Design review of the part built by this model. Coordinates are the model's own, in mm. A direction names the side the tool comes from. Coordinates: 2 decimals unless noted, no trailing zeros. Order: outer loops, then holes, each group sorted by start corner. A loop starts at its lowest first (then second) coordinate and runs counter-clockwise, first axis right, second up. Notation, with made-up numbers: (49.5, 11) -> (98.5, 11) arc R34 cw to (98.5, 41) -> close; hole circle Ø2 at (32.25, 79.5). An arc over 180 degrees is marked (long way). Use a Markdown table: item, result. Add a question column.
Q1. Add section C-C (z = 4). State the section outline as (x, y) points, then the cut area to 3 significant figures.
Q2. Machinability: for faces 1 (the face through (7.62, -3.16, 4.54)), 2 (the face through (-7, -5, 7)), 3 (the face through (-2.17, -9.76, 3.48)), which of the approach directions +Z, -Z, +X, -X, +Y, -Y give a long, thin tool a straight path to every point of the face, cutting with its end or side? Answer none if there is none.
Q3. Wall thickness on probe 1 along Y at (x, z) = (0, 3.4); probe 2 along Z at (x, y) = (2, -6); probe 3 along Y at (x, z) = (-5.5, 9.5): over which ranges is each line inside the solid? List them lowest first.
Q4. Insertion check: pin 1 (6 mm diameter, centred on x = -5.5, z = 3, fed in from +Y); pin 2 (4 mm diameter, centred on y = -3.5, z = 7.5, fed in from -X); pin 3 (2 mm diameter, centred on x = 1, z = 9, fed in from -Y). Each pin has a flat end and moves straight along its axis. Give the tip position at first contact, or say it passes through.
Q5. Add section A-A (y = 0). State the section outline as (x, z) points (3 decimals), then the cut area to 3 significant figures.
Q6. Add section D-D (z = 6). State the section outline as (x, y) points.
Q7. The part is to be moulded in two halves that separate along X. For faces 4 (the face through (4.449, -8.554, 8.576)), 5 (the face through (-1.978, -8.908, 8.331)), 6 (the face through (0, 0, 0)), say which applies: pulls with the +X half, pulls with the -X half, needs draft (parallel to the pull), parting line crosses it, or undercut.
from build123d import *

# Parameters (mm, degrees)
F0_R        = 10
F1_DEPTH    = 10
F2_R        = 8.25
F3_DEPTH    = 8
F4_R        = 9.125
F4_R_2      = 8.25
F5_DEPTH    = 3
F6_R        = 9.125
F6_R_2      = 8.75
F7_DEPTH    = 1
F8_R        = 2
F9_S5_R     = 9.125
F9_T6_DEPTH = 15
F10_SIZE2   = 5
F10_SIZE    = 0.5


# Not quite as in the source:
# - a fillet or chamfer that OpenCascade refuses, or shapes differently, is made with other operations: its cross-section is extruded or revolved along the edge and cut away or added


with BuildPart() as f1:
    # F0 (on Top) → F1 (new body)
    with BuildSketch(Plane.XY):
        Circle(F0_R)
    extrude(amount=F1_DEPTH)

    # F2 (on face) → F3 (cut)
    with BuildSketch(Plane.XY.offset(10)):
        Circle(F2_R)
    extrude(amount=-F3_DEPTH, mode=Mode.SUBTRACT)

    # F4 (on face) → F5 (cut)
    with BuildSketch(Plane.XY.offset(10)):
        Circle(F4_R)
        Circle(F4_R_2, mode=Mode.SUBTRACT)
    extrude(amount=-F5_DEPTH, mode=Mode.SUBTRACT)

    # F6 (on face) → F7 (join)
    with BuildSketch(Plane.XY.offset(10)):
        Circle(F6_R)
        Circle(F6_R_2, mode=Mode.SUBTRACT)
    extrude(amount=-F7_DEPTH)

    # F8
    f8_edges = [f1.edges().sort_by_distance(p)[0] for p in [
        (-10, 0, 0),
    ]]
    fillet(f8_edges, radius=F8_R)

    # F9: chamfer of 1 on 1 edges, made by hand


with BuildPart() as f9_tool2:
    # F9_s3 → F9_t4 (revolve)
    with BuildSketch(Plane.XZ):
        Polygon((8.75, 10), (9.75, 9), (8.75, 9), align=None)
    revolve(axis=Axis((0, 0, 9), (0, 0, 1)))

    # F9_s5 → F9_t6 (intersect, symmetric)
    with BuildSketch(Plane.XY.offset(9.5)):
        Circle(F9_S5_R)
    extrude(amount=F9_T6_DEPTH, both=True, mode=Mode.INTERSECT)


with BuildPart() as f1_1:
    add(f1.part)

    # F9_t1: cut F9_tool2
    add(f9_tool2.part, mode=Mode.SUBTRACT)

    # F10
    f10_edges = [f1_1.edges().sort_by_distance(p)[0] for p in [
        (-10, 0, 10),
    ]]
    f10_side = f1_1.faces().sort_by_distance((-9.717157, 0, 10))[0]
    chamfer(f10_edges, length=F10_SIZE, length2=F10_SIZE2, reference=f10_side)


solid = f1_1.part
Established:
| question | item | result |
|---|---|---|
| 1 | outline | circle Ø20 at (0, 0); hole circle Ø16.5 at (0, 0) |
| 1 | area | 100 mm^2 |
| 2 | face 1 | +Z |
| 2 | face 2 | none |
| 2 | face 3 | +Z, -Z |
| 3 | probe 1 | -10 to -8.25, 8.25 to 10 |
| 3 | probe 2 | 0 to 2 |
| 3 | probe 3 | -7.81 to -7.28, 7.28 to 7.81 |
| 4 | pin 1 | y = 9.68 |
| 4 | pin 2 | x = -9.69 |
| 4 | pin 3 | y = -9.67 |
| 5 | outline | (-10, 2) arc R2 ccw to (-8, 0) -> (8, 0) arc R2 ccw to (10, 2) -> (10, 5) -> (9.5, 10) -> (8.75, 10) -> (9.125, 9.625) -> (9.125, 7) -> (8.25, 7) -> (8.25, 2) -> (-8.25, 2) -> (-8.25, 7) -> (-9.125, 7) -> (-9.125, 9.625) -> (-8.75, 10) -> (-9.5, 10) -> (-10, 5) -> close |
| 5 | area | 58.7 mm^2 |
| 6 | outline | circle Ø19.8 at (0, 0); hole circle Ø16.5 at (0, 0) |
| 7 | face 4 | parting line crosses it |
| 7 | face 5 | undercut |
| 7 | face 6 | needs draft |
